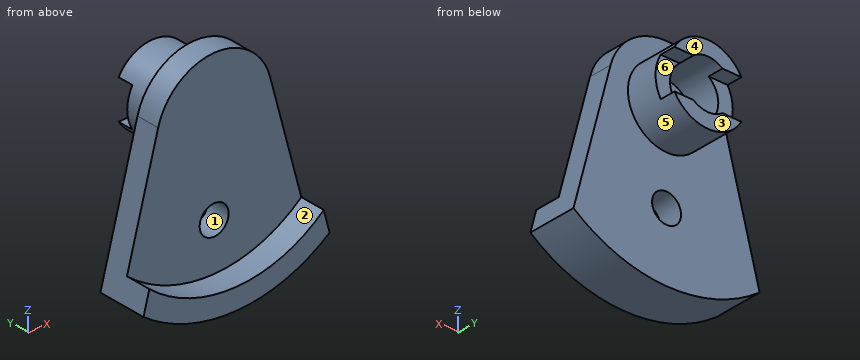
Autodesk Inventor part; units mm, degrees
ref_plane "YZ Plane" through (0, 0, 0) normal (1, 0, 0) x (0, 1, 0)
ref_plane "XZ Plane" through (0, 0, 0) normal (0, 1, 0) x (-1, 0, 0)
ref_plane "XY Plane" through (0, 0, 0) normal (0, 0, 1) x (1, 0, 0)
sketch "Sketch1" plane through (0, 0, 0) normal (0, 1, 0) x (-1, 0, 0)
  circle A0 centre (0, 0) radius 30
  circle A1 centre (0, 0) radius 20
  circle A2 centre (0, 0) radius 12.5
  line L0 (0, 0) -> (0, -45) construction
  circle A3 centre (0, -45) radius 7.5
  line L1 (-21, 10) -> (21, 10)
  line L2 (21, 10) -> (21, -10)
  line L3 (21, -10) -> (-21, -10)
  line L4 (-21, -10) -> (-21, 10)
  line L5 (-21, 10) -> (21, -10) construction
  line L6 (21, 10) -> (-21, -10) construction
  line L7 (28.9778, 7.7646) -> (48.1723, -63.8704)
  line L8 (-28.9778, 7.7646) -> (-48.1723, -63.8704)
  arc A4 (-48.1723, -63.8704) -> (48.1723, -63.8704) centre (0, 0) ccw
  arc A5 (-45.129, -52.5126) -> (45.129, -52.5126) centre (0, 0) ccw
  dimension "d0" = 60
  dimension "d1" = 40
  dimension "d2" = 25
  dimension "d5" = 45
  dimension "d6" = 15
  dimension "d7" = 42
  dimension "d8" = 20
  dimension "d11" = 80
  dimension "d12" = 30
  dimension "d13" = 15
  dimension "d19" = 69.2401
extrude "Extrusion1" add sketch "Sketch1" along normal blind 24 contours A1 L3 A2 L1 | L1 A2 A1 | A1 L3 A2 | L1 A2 L3 A1
extrude "Extrusion2" cut sketch "Sketch1" against normal blind 8 from surface at 24 contours A0 | A1 L3 A2 L1 | A1 L1 L2 L3 | L1 A2 L3 A1 | A1 L3 L4 L1 | A2 L3 L1
extrude "Extrusion3" add sketch "Sketch1" against normal blind 25 contours L7 A4 L8 A5
extrude "Extrusion4" add sketch "Sketch1" against normal blind 12 contours A0 | A0 L7 A5 L8 | A1 L3 A2 L1 | A1 L1 L2 L3 | L1 A2 A1 | A1 L3 A2 | L1 A2 L3 A1 | A1 L3 L4 L1 | L1 A2 | A2 L3 L1 | A2 L3
properties part number "C"
Could you check a few things on this model? Use its own coordinates, in mm. Face numbers are marked on the shaded views. A direction names the side the tool comes from. Give positions to 0.01 mm unless a question says otherwise; leave off trailing zeros. Write each loop counter-clockwise with the first axis right and the second up, starting at its lowest first coordinate (ties: lowest second). Pieces come first, ordered by that corner, then holes. Notation, with made-up numbers: (63.5, 28.5) - (103.5, 28.5) arc R13 cw to (103.5, 32.5) - close; hole circle Ø7 at (76.25, 46.25). An arc over 180 degrees is marked (long way). Use CSV: the item, a comma, the result in double quotes. Start each with the question number.
Item 1: I want a section at C-C, the plane y = 6. Please give me the cut outline in (x, z), then the cut area to 3 significant figures.
Item 2: For the marked faces 4, 5 and 6, which set-ups out of +Z, -Z, +X, -X, +Y, -Y let a thin tool reach every point of the face, with its end or its side?
Item 3: If I drill on line 1 along X through (y, z) = (12.5, 0); line 2 along Y through (x, z) = (-1, 8); line 3 along Z through (x, y) = (2, -3.5), over which ranges is the centre line in solid material (lowest first)?
Item 4: I want a section at A-A, the plane x = 0. Please give me the cut outline in (y, z).
Item 5: If we mould it in two halves opening along Z, with no side actions, what happens to the marked faces 1, 2 and 3? For each: pulls with the +Z half, pulls with the -Z half, needs draft (parallel to the pull), parting line crosses it, or undercut.
Item 6: I want a section at B-B, the plane z = -45. Please give me the cut outline in (x, y).
Item 7: I'm going to push flat-ended pins straight in: pin 1 (1 mm diameter, centred on x = -27, z = -16.5, fed in from -Y); pin 2 (8 mm diameter, centred on y = 6, z = -7, fed in from -X); pin 3 (4 mm diameter, centred on x = 11, y = 19.5, fed in from +Z); pin 4 (9 mm diameter, centred on x = 0, z = -45, fed in from +Y). Where does each tip first touch, or does it pass through?
Item 8: I want a section at D-D, the plane z = 16. Please give me the cut outline in (x, y).
Findings:
1,outline,"circle Ø40 at (0, 0); hole circle Ø25 at (0, 0)"
1,area,"766 mm2"
2,face 4,"+Z, -Z, +X, -X, +Y"
2,face 5,"+Y"
2,face 6,"+X, -X, +Y"
3,line 1,"x = -20 to -12.5, 12.5 to 20"
3,line 2,"y = -12 to 0"
3,line 3,"z = -79.97 to -52.23, -37.77 to 29.93"
4,outline,"(-25, -80) - (0, -80) - (0, -52.5) - (-12, -52.5) - (-12, -69.24) - (-25, -69.24) - close; (-12, -37.5) - (0, -37.5) - (0, -20) - (24, -20) - (24, -12.5) - (0, -12.5) - (0, 12.5) - (24, 12.5) - (24, 20) - (0, 20) - (0, 30) - (-12, 30) - close"
5,face 1,"undercut"
5,face 2,"pulls with the +Z half"
5,face 3,"needs draft"
6,outline,"(-43.12, -12) - (-7.5, -12) - (-7.5, 0) - (-43.12, 0) - close; (7.5, -12) - (43.12, -12) - (43.12, 0) - (7.5, 0) - close"
7,pin 1,"stops at y = -12"
7,pin 2,"stops at x = -19.77"
7,pin 3,"stops at z = 17.86"
7,pin 4,"passes through"
8,outline,"(-25.38, -12) - (25.38, -12) - (25.38, 0) - (12, 0) - (12, 24) - (-12, 24) - (-12, 0) - (-25.38, 0) - close"
